Geometry: final body of the model. Coordinates: model frame, mm. Round coordinates to 2 decimals unless told otherwise and drop trailing zeros. Loops run counter-clockwise (first coordinate to the right, second up) from the corner with the lowest first, then second, coordinate; pieces in that order, holes last. Notation, with made-up numbers: M 80.25,56 L 88.25,56 A23 ccw 88.25,78 Z; hole C 69.5,41 d10. An arc over 180 degrees is marked long. Write each question's results on one line, items separated by ' | '.
```python
from build123d import *

# Parameters (mm, degrees)
F1_DEPTH = 3.175
F2_W     = 3.175
F2_H     = 3.175
F3_DEPTH = 3.176


with BuildPart() as f1:
    # F0 (on Front) → F1 (new body)
    with BuildSketch(Plane.XZ):
        with BuildLine():
            Line((11.1704250392, 50.4924833011), (11.7423025331, 49.2882157063))
            ThreePointArc((11.7423025331, 49.2882157063), (11.4721766161, 49.8978586334), (11.1704250392, 50.4924833011))
        make_face()
        with BuildLine():
            Line((-11.1704250392, 50.4924833011), (11.1704250392, 50.4924833011))
            ThreePointArc((11.1704250392, 50.4924833011), (0, 57.15), (-11.1704250392, 50.4924833011))
        make_face()
        with BuildLine():
            ThreePointArc((-11.1704250392, 50.4924833011), (-11.4721766161, 49.8978586334), (-11.7423025331, 49.2882157063))
            Line((-11.7423025331, 49.2882157063), (-11.1704250392, 50.4924833011))
        make_face()
        with BuildLine():
            ThreePointArc((0, 31.75), (16.965239771, 26.8373459849), (28.6804415402, 13.6196465835))
            Line((28.6804415402, 13.6196465835), (11.7423025331, 49.2882157063))
            ThreePointArc((11.7423025331, 49.2882157063), (12.4582752051, 46.9160451972), (12.7, 44.45))
            ThreePointArc((12.7, 44.45), (8.9802561211, 35.4697438789), (0, 31.75))
        make_face()
        with BuildLine():
            Line((-11.7423025331, 49.2882157063), (-28.6804415402, 13.6196465835))
            ThreePointArc((-28.6804415402, 13.6196465835), (-16.965239771, 26.8373459849), (0, 31.75))
            ThreePointArc((0, 31.75), (-10.5530881611, 37.3844264023), (-11.7423025331, 49.2882157063))
        make_face()
        with BuildLine():
            ThreePointArc((-11.7423025331, 49.2882157063), (-10.5530881611, 37.3844264023), (0, 31.75))
            ThreePointArc((0, 31.75), (8.9802561211, 35.4697438789), (12.7, 44.45))
            ThreePointArc((12.7, 44.45), (12.4582752051, 46.9160451972), (11.7423025331, 49.2882157063))
            Line((11.7423025331, 49.2882157063), (11.1704250392, 50.4924833011))
            Line((11.1704250392, 50.4924833011), (-11.1704250392, 50.4924833011))
            Line((-11.1704250392, 50.4924833011), (-11.7423025331, 49.2882157063))
        make_face()
        with BuildLine():
            ThreePointArc((-28.6804415402, 13.6196465835), (-6.9806332485, -30.9731054215), (31.75, 0))
            ThreePointArc((31.75, 0), (30.9731054215, 6.9806332485), (28.6804415402, 13.6196465835))
            ThreePointArc((28.6804415402, 13.6196465835), (16.965239771, 26.8373459849), (0, 31.75))
            ThreePointArc((0, 31.75), (-16.965239771, 26.8373459849), (-28.6804415402, 13.6196465835))
        make_face()
    extrude(amount=F1_DEPTH)

    # F2 (on face) → F3 (cut, through all)
    with BuildSketch(Plane.XZ.offset(3.175)):
        Rectangle(F2_W, F2_H)
    extrude(amount=-F3_DEPTH, mode=Mode.SUBTRACT)


solid = f1.part
```
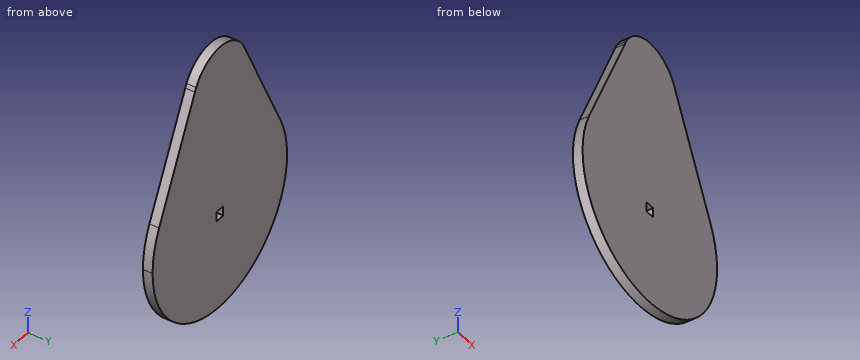
1. Section B-B (y = -0.55). Output: boundary loops of the cut face in (x, z).
Answer key:
outline: M -28.68,13.62 A31.75 ccw long 28.68,13.62 L 11.74,49.29 A12.7 ccw -11.74,49.29 Z; hole M -1.59,-1.59 L 1.59,-1.59 L 1.59,1.59 L -1.59,1.59 Z
2. Section D-D (z = -21). Output: boundary loops of the cut face in (x, y) (3 decimals), then the cut area to 3 significant figures.
Answer key:
outline: M -23.813,-3.175 L 23.813,-3.175 L 23.813,0 L -23.813,0 Z | area: 151 mm²
3. Ray query, probe 1 along X at (y, z) = (-3, 0.5); probe 2 along Z at (x, y) = (29, -1.6); probe 3 along Z at (x, y) = (7.5, -1.05). Return the intervals inside material, ascending.
Answer key:
probe 1: x = -31.75 to -1.59, 1.59 to 31.75 | probe 2: z = -12.93 to 12.93 | probe 3: z = -30.85 to 54.7
4. Section C-C (x = 18). Output: boundary loops of the cut face in (y, z) (3 decimals), then the cut area to 3 significant figures.
Answer key:
outline: M -3.175,-26.155 L 0,-26.155 L 0,36.111 L -3.175,36.111 Z | area: 198 mm²
